Geometry check sheet. Reference: the model listing, model coordinates, mm. A direction names the side the tool comes from. Give positions to 0.01 mm unless a question says otherwise; leave off trailing zeros. Loops run counter-clockwise (first coordinate to the right, second up) from the corner with the lowest first, then second, coordinate; pieces in that order, holes last. Notation, with made-up numbers: (-20, 13.25) -> (2, 13.25) arc R29 cw to (2, 48.25) -> close; hole circle Ø1 at (-14, -0.5). An arc over 180 degrees is marked (long way). Write item = value, one per line. Start each with the question number.
```python
from build123d import *

# Parameters (mm, degrees)
SKETCH_1_R      = 2.5
EXTRUDE_1_DEPTH = 4.5
SKETCH_2_R      = 4
SKETCH_2_R_2    = 2.5
EXTRUDE_2_DEPTH = 0.5
FILLET_1_R      = 0.2
FILLET_2_R      = 0.2


with BuildPart() as part:
    # 草图1 → 凸台-拉伸1 (new body)
    with BuildSketch(Plane.XY):
        Polygon((4.618802154, 0), (2.309401077, 4), (-2.309401077, 4), (-4.618802154, 0), (-2.309401077, -4), (2.309401077, -4), align=None)
        Circle(SKETCH_1_R, mode=Mode.SUBTRACT)
    extrude(amount=EXTRUDE_1_DEPTH)

    # 草图2 → 凸台-拉伸2 (add)
    with BuildSketch(Plane.XY.offset(4.5)):
        Circle(SKETCH_2_R)
        Circle(SKETCH_2_R_2, mode=Mode.SUBTRACT)
    extrude(amount=EXTRUDE_2_DEPTH)

    # 圆角1
    fillet_1_edges = [part.edges().sort_by_distance(p)[0] for p in [
        (-4, 0, 5),
    ]]
    fillet(fillet_1_edges, radius=FILLET_1_R)

    # 圆角2
    fillet_2_edges = [part.edges().sort_by_distance(p)[0] for p in [
        (0, -4, 0),
        (-3.464101615, -2, 0),
        (-3.464101615, 2, 0),
        (0, 4, 0),
        (3.464101615, 2, 0),
        (3.464101615, -2, 0),
    ]]
    fillet(fillet_2_edges, radius=FILLET_2_R)


solid = part.part
```
1) Depth check by flat-ended pin: pin 1 Ø2 at (x, z) = (3.5, 1) entering from -Y; pin 2 Ø3 at (x, y) = (0, 0) entering from -Z (3 decimals); pin 3 Ø2 at (y, z) = (1.5, 0.5) entering from -X. Enter the tip coordinate at first touch or a pass-through.
2) Thickness scan on line 1 (Y direction, x = 0, z = 1.55); line 2 (Y direction, x = 1.5, z = 1); line 3 (X direction, y = -1, z = 2.85). Record the ranges inside material, lowest first.
3) Tool access check on faces 1 (the flat face through (-2.1, -3.6, 4.5)), 2 (the flat face through (2.1, -3.6, 4.5)), 3 (the flat face through (-3.48, -1.97, 2.32)), 4 (the flat face through (-2.1, 3.6, 4.5)). Record the directions out of +Z, -Z, +X, -X, +Y, -Y that give a thin tool (end or side, any length) a straight path to the whole face; none if there is none.
4) Section check A-A (z = 2.5). Enter the section's corners in (x, y).
Check result:
q1.pin_1 = -3.67
q1.pin_2 = through
q1.pin_3 = -4.33
q2.line_1 = -4 to -2.5, 2.5 to 4
q2.line_2 = -4 to -2, 2 to 4
q2.line_3 = -4.04 to -2.29, 2.29 to 4.04
q3.face_1 = +Z, -X, -Y
q3.face_2 = +Z, +X, -Y
q3.face_3 = +Z, -Z, -X, -Y
q3.face_4 = +Z, -X, +Y
q4.outline = (-4.62, 0) -> (-2.31, -4) -> (2.31, -4) -> (4.62, 0) -> (2.31, 4) -> (-2.31, 4) -> close; hole circle Ø5 at (0, 0)
